Input: part model. Units: mm. Frame: model coordinates. A direction names the side the tool comes from. Coordinates: 2 decimals unless noted, no trailing zeros. Loops run counter-clockwise (first coordinate to the right, second up) from the corner with the lowest first, then second, coordinate; pieces in that order, holes last.
```python
from build123d import *

# Parameters (mm, degrees)
SKETCH_1_R      = 3.2
EXTRUDE_1_DEPTH = 6


with BuildPart() as part:
    # Эскиз1 → Бобышка-Вытянуть1 (new body)
    with BuildSketch(Plane(origin=(0, 0, 0), x_dir=(1, 0, 0), z_dir=(0, 1, 0))):
        Polygon((-27.603963146, 22.034878671), (-27.603963146, -27.965121329), (22.396036854, -27.965121329), (22.396036854, -22.965121329), (28.396036854, -22.965121329), (28.396036854, -12.965121329), (22.396036854, -12.965121329), (22.396036854, -4.365121329), (15.398535816, -4.365121329), (15.398739919, -5.764951191), (13.198739556, -5.765271964), (13.197678648, -4.364354869), (11.697679078, -4.365490812), (11.695559345, -1.566408326), (13.195558915, -1.565272383), (13.194498791, -0.165391578), (15.395321341, -0.165017325), (15.395559431, -1.565121329), (22.395560638, -1.565121329), (22.395560638, 7.034878671), (28.395560638, 7.034878671), (28.395560638, 17.034878671), (22.396036854, 17.034878671), (22.396036854, 22.034878671), (17.396036854, 22.034878671), (17.396036854, 28.034878671), (7.396036854, 28.034878671), (7.396036854, 22.034618289), (-1.203963146, 22.034810758), (-1.203963146, 15.03730972), (0.194846925, 15.037513675), (0.194793578, 12.837275467), (-1.206123677, 12.836452786), (-1.20524281, 11.336452446), (-4.003305339, 11.334809299), (-4.004186206, 12.834809041), (-5.40406717, 12.833986969), (-5.40406717, 15.034809551), (-4.003963146, 15.034809551), (-4.003963146, 22.034810758), (-12.603963146, 22.034878671), (-12.603963146, 28.034878671), (-22.603963146, 28.034878671), (-22.603963146, 22.034878671), align=None)
        with Locations((-2.603963146, -2.965121329)):
            Circle(SKETCH_1_R, mode=Mode.SUBTRACT)
    extrude(amount=EXTRUDE_1_DEPTH)


solid = part.part
```
Item 1: Contact query for flat-ended pins moving along their axis: P1, Ø1.8, axis at x = 19.5, y = 2.5, coming from the -Z side; P2, Ø2, axis at y = 5, z = 8, coming from the +X side; P3, Ø3, axis at y = 4, z = -26, coming from the -X side. Output: stop coordinate, or through.
Result:
P1: stops at z = -22.03
P2: stops at x = 22.4
P3: stops at x = -22.6
Item 2: Line query: L1, parallel to X at y = 3.1, z = -16; L2, parallel to Z at x = 15.5, y = 0.7; L3, parallel to Z at x = 20, y = 4.6. Output: solid intervals per line, ascending.
Result:
L1: x = -27.6 to -4, -1.2 to 28.4
L2: z = -28.03 to 1.57, 4.37 to 27.97
L3: z = -22.03 to 1.57, 4.37 to 27.97
Item 3: Section query C-C (x = -11.5). Output: boundary loops of the cut face in (y, z).
Result:
outline: (0, -22.03) - (6, -22.03) - (6, 27.97) - (0, 27.97) - close
Item 4: Section query D-D (z = 7.5). Output: boundary loops of the cut face in (x, y).
Result:
outline: (-27.6, 0) - (22.4, 0) - (22.4, 6) - (-27.6, 6) - close
Item 5: Section query B-B (z = -23.5). Output: boundary loops of the cut face in (x, y), then the cut area to 3 significant figures.
Result:
outline: (-22.6, 0) - (-12.6, 0) - (-12.6, 6) - (-22.6, 6) - close; (7.4, 0) - (17.4, 0) - (17.4, 6) - (7.4, 6) - close
area: 120 mm2
Item 6: Mould query, pull axis X, two halves, no side actions, for faces 5 (the face through (7.396, 3, -25)), 6 (the face through (22.396, 3, -19)), 7 (the face through (-22.604, 3, -25)). Classes: +X half, -X half, draft (parallel to the pull), parting line (faces both ways), or undercut.
Result:
face 5: undercut
face 6: +X half
face 7: -X half
Item 7: Section query A-A (x = 20.5). Output: boundary loops of the cut face in (y, z), then the cut area to 3 significant figures.
Result:
outline: (0, -22.03) - (6, -22.03) - (6, 1.57) - (0, 1.57) - close; (0, 4.37) - (6, 4.37) - (6, 27.97) - (0, 27.97) - close
area: 283 mm2
Item 8: Reachability of faces 1 (the face through (-5.404, 3, -14)), 2 (the face through (19, 3, 1.565)), 3 (the face through (-1.204, 3, -19)), 4 (the face through (22.396, 3, 26)) from +Z, -Z, +X, -X, +Y, -Y: full face, straight path, thin tool, end or side. Return the list, or none.
Result:
face 1: +Y, -Y
face 2: +X, +Y, -Y
face 3: -Z, +Y, -Y
face 4: +Z, +X, +Y, -Y
